Read the model definition and answer for the solid it produces. Units are mm, in the model's axes. A direction names the side the tool comes from. Round coordinates to 2 decimals unless told otherwise and drop trailing zeros. Order: outer loops, then holes, each group sorted by start corner. A loop starts at its lowest first (then second) coordinate and runs counter-clockwise, first axis right, second up. Notation, with made-up numbers: (-34.5, -10.75) -> (-26.5, -10.75) arc R10 ccw to (-26.5, -5.75) -> close; hole circle Ø11 at (31.25, 0.5). An arc over 180 degrees is marked (long way). Use a Markdown table: item, result. Add a question column.
1. Consider L1, parallel to X at y = 102, z = 11.25; L2, parallel to X at y = 109, z = 6; L3, parallel to X at y = 102.5, z = -1.5. Determine where each line is inside the solid, lowest interval first. Write a range as [from, to].
2. For faces 1 (the face through (74.1, 114.2, 6.858)), 2 (the face through (17.316, 139, 3)), 3 (the face through (17.316, 101, 3)), 4 (the face through (11.982, 124, 3)), 5 (the face through (15, 144.25, 3)), determine the directions among +Z, -Z, +X, -X, +Y, -Y from which every point of the face is accessible in a straight line to the end or side of a thin tool.
3. Section C-C, the plane z = -2 is taken. Give the vertices of the cut face in (x, y).
4. Given pin 1 (1 mm diameter, centred on y = 117.5, z = 4.5, fed in from +X); pin 2 (4 mm diameter, centred on x = 49.94, y = 102.21, fed in from -Z); pin 3 (10 mm diameter, centred on y = 144.5, z = 6, fed in from +X); pin 4 (5.5 mm diameter, centred on x = 13, y = 145, fed in from +Z), each flat-ended and moving along its own axis, determine where each tip first touches the part or whether it passes through.
5. Section B-B, the plane y = 123.5 is taken. Give the vertices of the cut face in (x, z), then the cut area to 3 significant figures.
6. Section A-A, the plane x = 76.2 is taken. Give the vertices of the cut face in (y, z), then the cut area to 3 significant figures.
7. Section D-D, the plane x = 59.5 is taken. Give the vertices of the cut face in (y, z), then the cut area to 3 significant figures.
8. The mould has two halves that part along X. Classify faces 6 (the face through (17.316, 133, 3)), 7 (the face through (56.537, 111, 0)), 8 (the face through (52, 125.2, 5)): +X half, -X half, draft (parallel to the pull), parting line (faces both ways), or undercut.
```python
from build123d import *

# Parameters (mm, degrees)
BOSS_EXTRUDE1_DEPTH = 6.858
SKETCH3_R           = 2.54
SKETCH3_R_2         = 3.77436477
BOSS_EXTRUDE2_DEPTH = 5.08
SKETCH4_R           = 2.54
BOSS_EXTRUDE3_DEPTH = 13.97


with BuildPart() as part:
    # Sketch2 → Boss-Extrude1 (new body)
    with BuildSketch(Plane.XY):
        Polygon((11.982344641, 125.199618103), (11.982344641, 121.897618103), (17.316344641, 121.897618103), (17.316344641, 118.849618103), (11.982344641, 118.849618103), (11.982344641, 115.547618103), (17.316344641, 115.547618103), (17.316344641, 112.499618103), (11.982344641, 112.499618103), (11.982344641, 109.197618103), (17.316344641, 109.197618103), (17.316344641, 106.149618103), (11.982344641, 106.149618103), (11.982344641, 102.847618103), (17.316344641, 102.847618103), (17.316344641, 99.799618103), (11.982344641, 99.799618103), (11.982344641, 96.497618103), (6.729436841, 96.497618103), (6.729436841, 125.199618103), (6.729436841, 150.218618103), (11.982344641, 150.218618103), (11.982344641, 147.297618103), (17.316344641, 147.297618103), (17.316344641, 144.249618103), (11.982344641, 144.249618103), (11.982344641, 140.947618103), (17.316344641, 140.947618103), (17.316344641, 137.899618103), (11.982344641, 137.899618103), (11.982344641, 134.597618103), (17.316344641, 134.597618103), (17.316344641, 131.549618103), (11.982344641, 131.549618103), (11.982344641, 128.247618103), (17.316344641, 128.247618103), (17.316344641, 125.199618103), align=None)
    extrude(amount=BOSS_EXTRUDE1_DEPTH)

    # Sketch3 → Boss-Extrude2 (add)
    with BuildSketch(Plane.XY.offset(6.858)):
        with BuildLine():
            Line((6.729436841, 125.199618103), (6.729436841, 96.497618103))
            Line((6.729436841, 96.497618103), (16.3439883, 96.497618103))
            Line((16.3439883, 96.497618103), (32.312638487, 96.497618103))
            Line((32.312638487, 96.497618103), (78.23353946, 96.497618103))
            Line((78.23353946, 96.497618103), (92.175808331, 96.497618103))
            Line((92.175808331, 96.497618103), (92.175808331, 125.199618103))
            Line((92.175808331, 125.199618103), (78.23353946, 125.199618103))
            Line((78.23353946, 125.199618103), (36.33380561, 125.199618103))
            ThreePointArc((36.33380561, 125.199618103), (32.5002138, 125.792034783), (29.024272972, 127.514015924))
            Line((29.024272972, 127.514015924), (6.729436841, 143.205434636))
            Line((6.729436841, 143.205434636), (6.729436841, 125.199618103))
        make_face()
        with Locations((24.539097495, 102.212466287)):
            Circle(SKETCH3_R, mode=Mode.SUBTRACT)
        with Locations((76.2, 110.848618103)):
            Circle(SKETCH3_R_2, mode=Mode.SUBTRACT)
        with Locations((24.539097495, 119.484769918)):
            Circle(SKETCH3_R, mode=Mode.SUBTRACT)
        with Locations((37.239097495, 119.484769918)):
            Circle(SKETCH3_R, mode=Mode.SUBTRACT)
        with Locations((37.239097495, 102.212466287)):
            Circle(SKETCH3_R, mode=Mode.SUBTRACT)
        with Locations((49.939097495, 119.484769918)):
            Circle(SKETCH3_R, mode=Mode.SUBTRACT)
        with Locations((49.939097495, 102.212466287)):
            Circle(SKETCH3_R, mode=Mode.SUBTRACT)
    extrude(amount=BOSS_EXTRUDE2_DEPTH)

    # Sketch4 → Boss-Extrude3 (add)
    with BuildSketch(Plane(origin=(0, 0, 6.858), x_dir=(-1, 0, 0), z_dir=(0, 0, -1))):
        with BuildLine():
            Line((-29.024272972, 127.514015924), (-18.664038362, 134.805694511))
            Line((-18.664038362, 134.805694511), (-18.664038362, 96.497618103))
            Line((-18.664038362, 96.497618103), (-56.536837783, 96.497618103))
            Line((-56.536837783, 96.497618103), (-56.536837783, 125.199618103))
            Line((-56.536837783, 125.199618103), (-36.33380561, 125.199618103))
            ThreePointArc((-36.33380561, 125.199618103), (-32.5002138, 125.792034783), (-29.024272972, 127.514015924))
        make_face()
        with Locations((-49.939097495, 102.212466287)):
            Circle(SKETCH4_R, mode=Mode.SUBTRACT)
        with Locations((-37.239097495, 102.212466287)):
            Circle(SKETCH4_R, mode=Mode.SUBTRACT)
        with Locations((-24.539097495, 102.212466287)):
            Circle(SKETCH4_R, mode=Mode.SUBTRACT)
        with Locations((-24.539097495, 119.484769918)):
            Circle(SKETCH4_R, mode=Mode.SUBTRACT)
        with Locations((-37.239097495, 119.484769918)):
            Circle(SKETCH4_R, mode=Mode.SUBTRACT)
        with Locations((-49.939097495, 119.484769918)):
            Circle(SKETCH4_R, mode=Mode.SUBTRACT)
    extrude(amount=BOSS_EXTRUDE3_DEPTH)


solid = part.part
```
Verdict:
| question | item | result |
|---|---|---|
| 1 | L1 | x = [6.73, 22.01], [27.07, 34.71], [39.77, 47.41], [52.47, 92.18] |
| 1 | L2 | x = [6.73, 17.32], [18.66, 56.54] |
| 1 | L3 | x = [18.66, 22.02], [27.06, 34.72], [39.76, 47.42], [52.46, 56.54] |
| 2 | face 1 | -Z, +X, +Y, -Y |
| 2 | face 2 | +Z, -Z, +X, +Y, -Y |
| 2 | face 3 | -Z, +Y, -Y |
| 2 | face 4 | -Z |
| 2 | face 5 | +Z, -Z, +X |
| 3 | outline | (18.66, 96.5) -> (56.54, 96.5) -> (56.54, 125.2) -> (36.33, 125.2) arc R12.7 cw to (29.02, 127.51) -> (18.66, 134.81) -> close; hole circle Ø5.08 at (24.54, 102.21); hole circle Ø5.08 at (24.54, 119.48); hole circle Ø5.08 at (37.24, 102.21); hole circle Ø5.08 at (37.24, 119.48); hole circle Ø5.08 at (49.94, 102.21); hole circle Ø5.08 at (49.94, 119.48) |
| 4 | pin 1 | stops at x = 56.54 |
| 4 | pin 2 | passes through |
| 4 | pin 3 | stops at x = 17.32 |
| 4 | pin 4 | stops at z = 6.86 |
| 5 | outline | (6.73, 0) -> (11.98, 0) -> (11.98, 6.86) -> (18.66, 6.86) -> (18.66, -7.11) -> (56.54, -7.11) -> (56.54, 6.86) -> (92.18, 6.86) -> (92.18, 11.94) -> (6.73, 11.94) -> close |
| 5 | area | 999 mm2 |
| 6 | outline | (96.5, 6.86) -> (107.07, 6.86) -> (107.07, 11.94) -> (96.5, 11.94) -> close; (114.62, 6.86) -> (125.2, 6.86) -> (125.2, 11.94) -> (114.62, 11.94) -> close |
| 6 | area | 107 mm2 |
| 7 | outline | (96.5, 6.86) -> (125.2, 6.86) -> (125.2, 11.94) -> (96.5, 11.94) -> close |
| 7 | area | 146 mm2 |
| 8 | face 6 | undercut |
| 8 | face 7 | +X half |
| 8 | face 8 | draft |
